from build123d import *

# Parameters (mm, degrees)
F0_R     = 3.975
F1_DEPTH = 25
F2_DEPTH = 4
F3_SIZE  = 1


with BuildPart() as f1:
    # F0 (on Top) → F1 (new body)
    with BuildSketch(Plane.XY):
        with Locations((-61.589289, -9.165525)):
            Circle(F0_R)
    extrude(amount=F1_DEPTH)

    # F0 (on Top) → F2 (join)
    with BuildSketch(Plane.XY):
        Polygon((-61.685733, -17.164943), (-54.709811, -13.248756), (-54.613368, -5.249337), (-61.492846, -1.166106), (-68.468768, -5.082293), (-68.565211, -13.081712), align=None)
        with Locations((-61.589289, -9.165525)):
            Circle(F0_R, mode=Mode.SUBTRACT)
    extrude(amount=F2_DEPTH)

    # F3
    f3_edges = [f1.edges().sort_by_distance(p)[0] for p in [
        (-65.125472, -15.123327, 0),
        (-58.197772, -15.20685, 0),
        (-54.66159, -9.249047, 0),
        (-58.053107, -3.207722, 0),
        (-64.980807, -3.124199, 0),
        (-68.516989, -9.082002, 0),
    ]]
    chamfer(f3_edges, length=F3_SIZE)


solid = f1.part
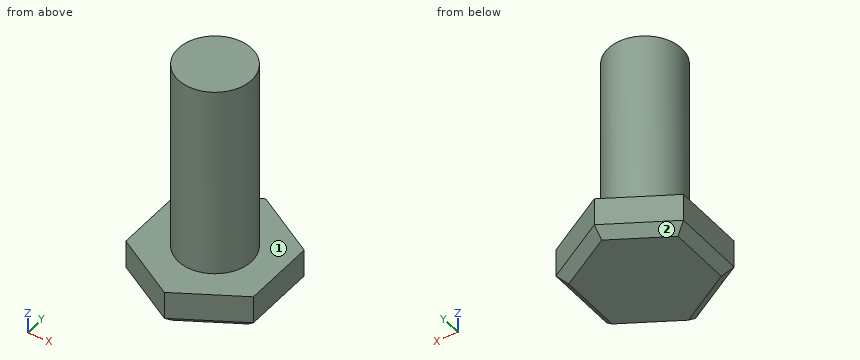
CAD build for the part. Positions are in the model's coordinates, mm. Face numbers are marked on the shaded views. A direction names the side the tool comes from. Round coordinates to 2 decimals unless told otherwise and drop trailing zeros. Write each loop counter-clockwise with the first axis right and the second up, starting at its lowest first coordinate (ties: lowest second). Pieces come first, ordered by that corner, then holes. Notation, with made-up numbers: (-34, 51.5) -> (22, 51.5) arc R16 cw to (22, 62.5) -> close; hole circle Ø6 at (28.5, 89.5). An arc over 180 degrees is marked (long way). Answer as a JSON object with one key per item and string values.
(1) Band-saw the part on B-B, the plane y = -7. List the corners of the cut face in (x, z), then the cut area to 3 significant figures.
Reported:
{"outline": "(-68.49, 1) -> (-67.49, 0) -> (-55.63, 0) -> (-54.63, 1) -> (-54.63, 4) -> (-58.26, 4) -> (-58.26, 25) -> (-64.92, 25) -> (-64.92, 4) -> (-68.49, 4) -> close", "area": "194 mm^2"}
(2) Band-saw the part on A-A, the plane x = -58. List the corners of the cut face in (y, z), then the cut area to 3 significant figures.
Reported:
{"outline": "(-15.1, 1) -> (-13.95, 0) -> (-4.4, 0) -> (-3.24, 1) -> (-3.24, 4) -> (-7.46, 4) -> (-7.46, 25) -> (-10.87, 25) -> (-10.87, 4) -> (-15.1, 4) -> close", "area": "118 mm^2"}
(3) Which spindle directions (+Z, -Z, +X, -X, +Y, -Y) get a long thin tool onto all of the face, cutting with end or side? Do the marked faces 1 and 2. Say none if no direction does.
Reported:
{"face 1": "+Z", "face 2": "-Z, -X, +Y"}
(4) Band-saw the part on D-D, the plane x = -67. List the corners of the cut face in (y, z), then the cut area to 3 significant figures.
Reported:
{"outline": "(-14.01, 1) -> (-12.85, 0) -> (-5.4, 0) -> (-4.26, 1) -> (-4.26, 4) -> (-14.01, 4) -> close", "area": "37.9 mm^2"}
(5) Band-saw the part on C-C, the plane y = -2.75. List the corners of the cut face in (x, z).
Reported:
{"outline": "(-64.31, 1) -> (-62.27, 0) -> (-60.78, 0) -> (-58.82, 1) -> (-58.82, 4) -> (-64.31, 4) -> close"}
(6) Pin check, flat tips, straight feed: P1, Ø4, axis at y = -10.5, z = 11.5, coming from the +X side; P2, Ø1, axis at x = -60, z = 3, coming from the -Y side; P3, Ø5, axis at x = -60.5, y = -5, coming from the +Z side; P4, Ø1.5, axis at x = -59.5, z = 9, coming from the +Y side. Stop position of each tip, or through.
Reported:
{"P1": "stops at x = -57.61", "P2": "stops at y = -16.5", "P3": "stops at z = 25", "P4": "stops at y = -5.42"}
(7) Probe probe 1 along Z at (x, y) = (-55.75, -11.5); probe 2 along X at (y, z) = (-9, 17); probe 3 along Y at (x, z) = (-62.25, 6.25). List the from-to ranges inside material, lowest first. Write a range as [from, to].
Reported:
{"probe 1": "z = [0, 4]", "probe 2": "x = [-65.56, -57.62]", "probe 3": "y = [-13.09, -5.25]"}
